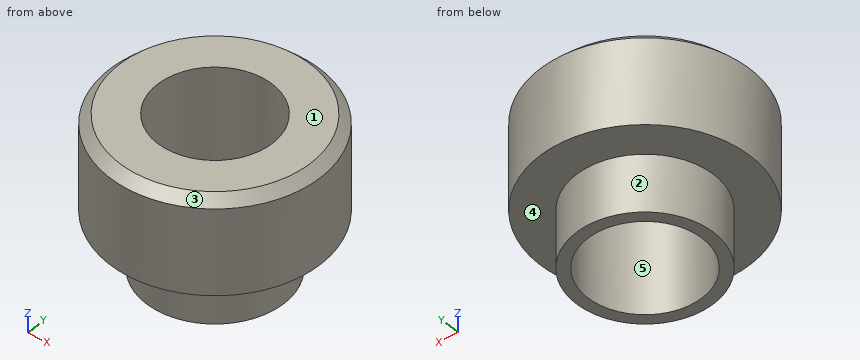
Autodesk Inventor part; units mm, degrees
ref_plane "YZ Plane" through (0, 0, 0) normal (1, 0, 0) x (0, 1, 0)
ref_plane "XZ Plane" through (0, 0, 0) normal (0, 1, 0) x (-1, 0, 0)
ref_plane "XY Plane" through (0, 0, 0) normal (0, 0, 1) x (1, 0, 0)
sketch "Эскиз1" plane through (0, 0, 0) normal (0, 1, 0) x (-1, 0, 0)
  line L0 (0, 0) -> (2.75, 0)
  line L1 (2.75, 0) -> (2.75, 2.5)
  line L2 (2.75, 2.5) -> (-2.75, 2.5)
  line L3 (-2.75, 2.5) -> (-2.75, 0)
  line L4 (-2.75, 0) -> (2.75, 0)
  line L5 (0, 0) -> (1.8, 0)
  line L6 (1.8, 0) -> (1.8, -1.5)
  line L7 (1.8, -1.5) -> (-1.8, -1.5)
  line L8 (-1.8, -1.5) -> (-1.8, 0)
  line L9 (0, 2.5) -> (1.5, 2.5)
  line L10 (1.5, 2.5) -> (1.5, -1.5)
  line L11 (0, -1.5) -> (0, 2.5)
  dimension "d0" = 2.75
  dimension "d1" = 2.5
  dimension "d2" = 5.5
  dimension "d3" = 1.8
  dimension "d4" = 1.5
  dimension "d5" = 3.6
  dimension "d6" = 1.5
revolve "Вращение1" add sketch "Эскиз1" angle 360 about axis through (0, 0, -1.5) along (0, 0, 1) contours L0 L10 L2 L1 | L6 L7 L10 L0
thread "Резьба1"
chamfer "Фаска1" distance 0.25 angle 45 1 edges at (2.75, 0, 2.5)
properties part number "soldered nut"
The listing builds one solid part. Answer for the finished solid, in the listing's coordinates (mm). Face numbers are marked on the shaded views. A direction names the side the tool comes from. Coordinates: 2 decimals unless noted, no trailing zeros. Write each loop counter-clockwise with the first axis right and the second up, starting at its lowest first coordinate (ties: lowest second). Pieces come first, ordered by that corner, then holes. Notation, with made-up numbers: M -28.75,-37 L 0.25,-37 A28 ccw 0.25,-4 Z; hole C -15.5,56 d2. An arc over 180 degrees is marked long. Put each result on its own line as item: value. Start each with the question number.
1. Flat-ended cylindrical pins translate along their axes: P1, Ø1.5, axis at x = 1, y = -0.5, coming from the -Z side; P2, Ø1.5, axis at x = -1, z = -1, coming from the +Y side; P3, Ø1, axis at x = -1, z = 0, coming from the +Y side. Find the tip coordinate at first contact, or state that the pin passes through.
2. A cutting plane is placed at C-C on z = -0.2. Write down the section's boundary in (x, y), then the cut area to 3 significant figures.
3. Which of the six approach directions +Z, -Z, +X, -X, +Y, -Y give full straight-line access (tool end or side, diameter ignored) to the marked faces 1 and 2?
4. Consider line 1 (X direction, y = 0, z = 1); line 2 (Y direction, x = 0, z = -0.4). Determine where each line is inside the solid, lowest interval first. Write a range as from..to.
5. A cutting plane is placed at A-A on x = 0. Write down the section's boundary in (y, z), then the cut area to 3 significant figures.
6. A cutting plane is placed at D-D on z = 0.6. Write down the section's boundary in (x, y), then the cut area to 3 significant figures.
7. For a pull along X with two mould halves and no side action, classify the marked faces 3, 4 and 5 as pulls with the +X half, pulls with the -X half, needs draft (parallel to the pull), parting line crosses it, or undercut.
Resolved:
1. P1: stops at z = -1.5
1. P2: stops at y = 1.78
1. P3: stops at y = 2.7
2. outline: C 0,0 d3.6; hole C 0,0 d3
2. area: 3.11 mm2
3. face 1: +Z, +X, -X, +Y, -Y
3. face 2: -Z
4. line 1: x = -2.75..-1.5, 1.5..2.75
4. line 2: y = -1.8..-1.5, 1.5..1.8
5. outline: M -2.75,0 L -1.8,0 L -1.8,-1.5 L -1.5,-1.5 L -1.5,2.5 L -2.5,2.5 L -2.75,2.25 Z; M 1.5,-1.5 L 1.8,-1.5 L 1.8,0 L 2.75,0 L 2.75,2.25 L 2.5,2.5 L 1.5,2.5 Z
5. area: 7.09 mm2
6. outline: C 0,0 d5.5; hole C 0,0 d3
6. area: 16.7 mm2
7. face 3: parting line crosses it
7. face 4: needs draft
7. face 5: undercut
